Verification items for this drawing (mm, ordinates from the low corner). A direction names the side the tool comes from. Coordinates: 2 decimals unless noted, no trailing zeros. Order: outer loops, then holes, each group sorted by start corner. A loop starts at its lowest first (then second) coordinate and runs counter-clockwise, first axis right, second up.
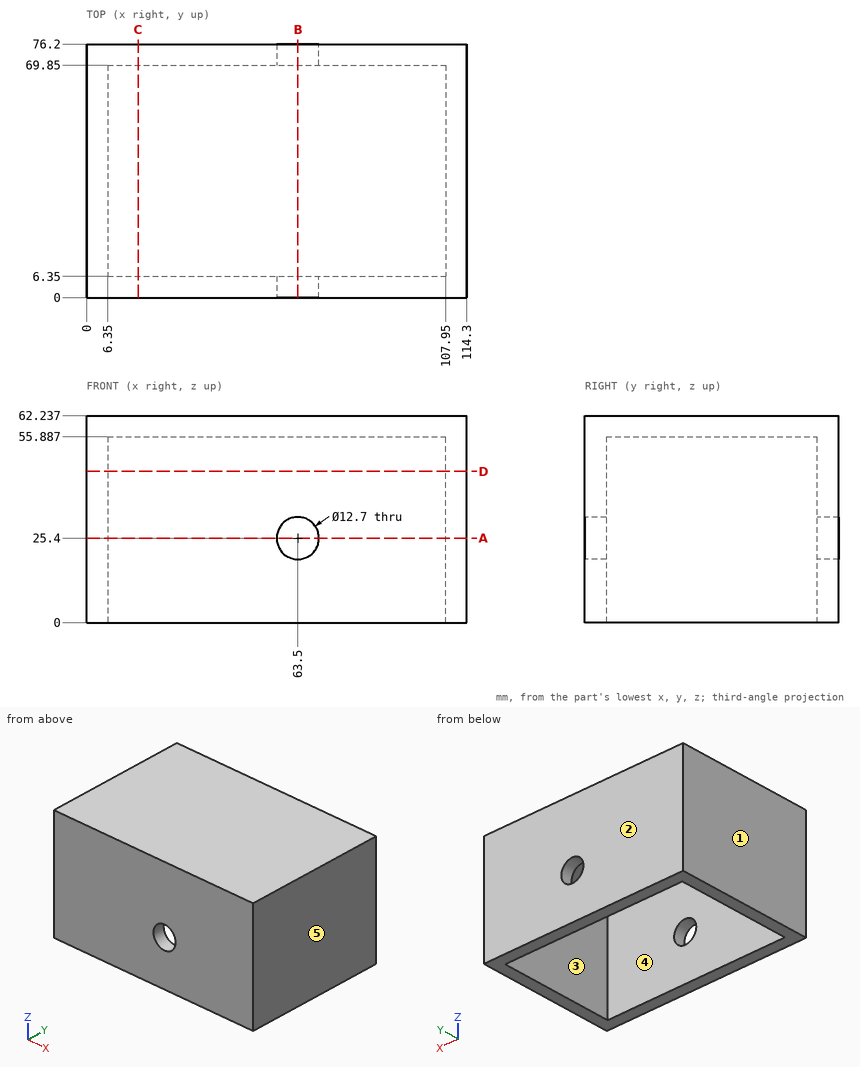
Item 1: Sectioned sample at B-B (x = 63.5). Record the cut outline in (y, z).
Item 2: Sectioned sample at A-A (z = 25.4). Record the cut outline in (x, y).
Item 3: Tool access check on the marked faces 4 and 5. Record the directions out of +Z, -Z, +X, -X, +Y, -Y that give a thin tool (end or side, any length) a straight path to the whole face; none if there is none.
Item 4: Release check for a two-part mould opening along X. For the marked faces 1, 2 and 3 record: pulls with the +X half, pulls with the -X half, needs draft (parallel to the pull), parting line crosses it, or undercut.
Item 5: Depth check by flat-ended pin: P1, Ø20.5, axis at x = 63.5, z = 25.4, coming from the -Y side. Enter the tip coordinate at first touch or a pass-through.
Item 6: Sectioned sample at C-C (x = 15.5). Record the cut outline in (y, z).
Item 7: Sectioned sample at D-D (z = 45.5). Record the cut outline in (x, y), and give its area (3 significant figures).
Item 8: Thickness scan on line 1 along Y through (x, z) = (86, 12.5); line 2 along X through (y, z) = (25.5, 7.5); line 3 along Z through (x, y) = (63.5, 71.5). Record the ranges inside material, lowest first.
Geometry check:
1. outline: (0, 0) - (6.35, 0) - (6.35, 19.05) - (0, 19.05) - close; (0, 31.75) - (6.35, 31.75) - (6.35, 55.89) - (69.85, 55.89) - (69.85, 31.75) - (76.2, 31.75) - (76.2, 62.24) - (0, 62.24) - close; (69.85, 0) - (76.2, 0) - (76.2, 19.05) - (69.85, 19.05) - close
2. outline: (0, 0) - (57.15, 0) - (57.15, 6.35) - (6.35, 6.35) - (6.35, 69.85) - (57.15, 69.85) - (57.15, 76.2) - (0, 76.2) - close; (69.85, 0) - (114.3, 0) - (114.3, 76.2) - (69.85, 76.2) - (69.85, 69.85) - (107.95, 69.85) - (107.95, 6.35) - (69.85, 6.35) - close
3. face 4: -Z
3. face 5: +Z, -Z, +X, +Y, -Y
4. face 1: pulls with the -X half
4. face 2: needs draft
4. face 3: undercut
5. P1: stops at y = 0
6. outline: (0, 0) - (6.35, 0) - (6.35, 55.89) - (69.85, 55.89) - (69.85, 0) - (76.2, 0) - (76.2, 62.24) - (0, 62.24) - close
7. outline: (0, 0) - (114.3, 0) - (114.3, 76.2) - (0, 76.2) - close; hole (6.35, 6.35) - (107.95, 6.35) - (107.95, 69.85) - (6.35, 69.85) - close
7. area: 2,260 mm2
8. line 1: y = 0 to 6.35, 69.85 to 76.2
8. line 2: x = 0 to 6.35, 107.95 to 114.3
8. line 3: z = 0 to 19.05, 31.75 to 62.24
